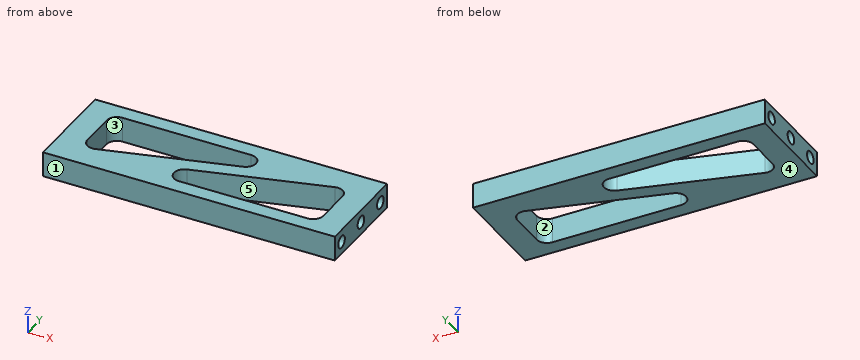
Autodesk Inventor part; units mm, degrees
ref_plane "YZ Plane" through (0, 0, 0) normal (1, 0, 0) x (0, 1, 0)
ref_plane "XZ Plane" through (0, 0, 0) normal (0, 1, 0) x (-1, 0, 0)
ref_plane "XY Plane" through (0, 0, 0) normal (0, 0, 1) x (1, 0, 0)
sketch "スケッチ1" plane through (0, 0, 0) normal (0, 0, 1) x (1, 0, 0)
  line L0 (-29.15, 9.75) -> (29.15, 9.75)
  line L1 (29.15, 9.75) -> (29.15, -9.75)
  line L2 (29.15, -9.75) -> (-29.15, -9.75)
  line L3 (-29.15, -9.75) -> (-29.15, 9.75)
  line L4 (-24.15, 6.75) -> (24.15, 6.75) construction
  line L5 (24.15, 6.75) -> (24.15, -6.75) construction
  line L6 (24.15, -6.75) -> (-24.15, -6.75) construction
  line L7 (-24.15, -6.75) -> (-24.15, 6.75) construction
  line L8 (24.15, 6.75) -> (-24.15, -6.75) construction
  line L9 (-24.15, -5.1925) -> (-24.15, 6.75)
  line L10 (-24.15, 6.75) -> (18.5776, 6.75)
  line L11 (18.5776, 6.75) -> (-24.15, -5.1925)
  line L12 (-18.5776, -6.75) -> (24.15, -6.75)
  line L13 (24.15, -6.75) -> (24.15, 5.1925)
  line L14 (24.15, 5.1925) -> (-18.5776, -6.75)
  line L15 (-29.15, 7.25) -> (29.15, 7.25) construction
  line L16 (29.15, -7.25) -> (-29.15, -7.25) construction
  line L17 (29.15, 7.25) -> (29.15, -7.25) construction
  point P0 (0, 0)
  point P1 (0, 6.75)
  point P2 (0, 9.75)
  point P3 (24.15, 0)
  point P4 (29.15, 0)
  dimension "d0" = 5
  dimension "d1" = 3
  dimension "d2" = 1.5
  dimension "d3" = 14.5
  dimension "d4" = 2.5
  dimension "d16" = 58.3
extrude "押し出し1" add sketch "スケッチ1" along normal blind 5
sketch "スケッチ2" plane through (29.15, -9.75, 0) normal (1, 0, 0) x (0, 0, -1)
  line L0 (0, 19.5) -> (-5, 19.5)
  line L1 (-5, 0) -> (-5, 19.5)
  line L2 (0, 9.75) -> (-5, 9.75) construction
  point P0 (-2.5, 2.5)
  point P1 (-2.5, 9.75)
  point P2 (-2.5, 17)
  point P3 (-2.5, 19.5)
  dimension "d7" = 14.5
hole "穴1" at (29.15, -7.25, 2.5) at (29.15, 7.25, 2.5) at (29.15, 0, 2.5) direction (-1, 0, 0) diameter 2.459 depth 3
mirror "ミラー1" about plane through (0, 0, 0) normal (1, 0, 0) of "穴1"
fillet "フィレット3" radius 2.05 6 edges at (-24.15, 6.75, 2.5) (18.5776, 6.75, 2.5) (24.15, 5.1925, 2.5) (24.15, -6.75, 2.5) (-18.5776, -6.75, 2.5) (-24.15, -5.1925, 2.5)
properties part number "リンク_ふくらはぎ_サブフレーム_1_2(予備案)" material "アルミニウム 2014-T4"
Could you check a few things on this model? Use its own coordinates, in mm. Face numbers are marked on the shaded views. A direction names the side the tool comes from. Coordinates: 2 decimals unless noted, no trailing zeros. Order: outer loops, then holes, each group sorted by start corner. A loop starts at its lowest first (then second) coordinate and runs counter-clockwise, first axis right, second up. Notation, with made-up numbers: (19.5, 33) -> (74.5, 33) arc R23 cw to (74.5, 50) -> close; hole circle Ø1 at (-20, 42). An arc over 180 degrees is marked (long way). One line per question, with ' | ' between items.
Q1. Imagine slicing it at A-A on x = -7.5. Please give me the cut outline in (y, z).
Return value:
outline: (-9.75, 0) -> (-0.54, 0) -> (-0.54, 5) -> (-9.75, 5) -> close; (6.75, 0) -> (9.75, 0) -> (9.75, 5) -> (6.75, 5) -> close
Q2. Imagine slicing it at D-D on z = 2.5. State how many separate pieces and enclosed holes the cut face has, and give its area (3 significant figures).
Return value:
separate pieces: 1 | enclosed holes: 2 | area: 637 mm²
Q3. I'm going to push flat-ended pins straight in: P1, Ø0.7, axis at y = 0, z = 2.5, coming from the +X side; P2, Ø0.7, axis at y = -0.5, z = 3, coming from the -X side; P3, Ø3, axis at x = -21, y = 2, coming from the -Z side. Where does each tip first touch, or does it pass through?
Return value:
P1: x = 26.15 | P2: x = -26.15 | P3: through
Q4. If I drill on L1, parallel to Y at x = -27.8, z = 2.5; L2, parallel to Z at x = -27.75, y = 0; L3, parallel to Y at x = 14.5, z = 1.05, over which ranges is the centre line in solid material (lowest first)?
Return value:
L1: -9.75 to -8.48, -6.02 to -1.23, 1.23 to 6.02, 8.48 to 9.75 | L2: 0 to 1.27, 3.73 to 5 | L3: -9.75 to -6.75, 2.5 to 9.75
Q5. Imagine slicing it at B-B on x = 2. Please give me the cut outline in (y, z).
Return value:
outline: (-9.75, 0) -> (-6.75, 0) -> (-6.75, 5) -> (-9.75, 5) -> close; (-1, 0) -> (2.12, 0) -> (2.12, 5) -> (-1, 5) -> close; (6.75, 0) -> (9.75, 0) -> (9.75, 5) -> (6.75, 5) -> close
Q6. On a 3-axis mill with a long thin cutter (end or side, diameter ignored), from which of +Z, -Z, +X, -X, +Y, -Y can I reach the whole of each face in a straight line? I mean the marked faces 1 and 2. Say none if no direction works.
Return value:
face 1: +Z, -Z, +X, -X, -Y | face 2: +Z, -Z
Q7. Thinking about a two-plate mould opening in X: for the marked faces 3, 4 and 5, which applies, pulls with the +X half, pulls with the -X half, needs draft (parallel to the pull), parting line crosses it, or undercut?
Return value:
face 3: undercut | face 4: needs draft | face 5: undercut
Q8. Imagine slicing it at C-C on y = 0. Please give me the cut outline in (x, z).
Return value:
outline: (-29.15, 0) -> (-24.15, 0) -> (-24.15, 5) -> (-29.15, 5) -> (-29.15, 3.73) -> (-26.15, 3.73) -> (-26.15, 1.27) -> (-29.15, 1.27) -> close; (-5.57, 0) -> (5.57, 0) -> (5.57, 5) -> (-5.57, 5) -> close; (24.15, 0) -> (29.15, 0) -> (29.15, 1.27) -> (26.15, 1.27) -> (26.15, 3.73) -> (29.15, 3.73) -> (29.15, 5) -> (24.15, 5) -> close
